```python
from build123d import *

# Parameters (mm, degrees)
BOSS_EXTRUDE1_DEPTH            = 3.175
M2X0_4_TAPPED_HOLE1_AT_2_COUNT = 2
M2X0_4_TAPPED_HOLE1_AT_2_PITCH = 18.662705418
CIRPATTERN1_COUNT              = 6


with BuildPart() as part:
    # Sketch1 → Boss-Extrude1 (new body)
    with BuildSketch(Plane(origin=(0, 0, 0), x_dir=(1, 0, 0), z_dir=(0, 1, 0))):
        Polygon((60.998522628, 0), (30.499261314, 52.826270189), (-30.499261314, 52.826270189), (-60.998522628, 0), (-30.499261314, -52.826270189), (30.499261314, -52.826270189), align=None)
        with BuildLine():
            Line((52.749630657, 1.5875), (27.749630657, 44.888770189))
            ThreePointArc((27.749630657, 44.888770189), (26.5875, 46.050900846), (25, 46.476270189))
            Line((25, 46.476270189), (-25, 46.476270189))
            ThreePointArc((-25, 46.476270189), (-26.5875, 46.050900846), (-27.749630657, 44.888770189))
            Line((-27.749630657, 44.888770189), (-52.749630657, 1.5875))
            ThreePointArc((-52.749630657, 1.5875), (-53.175, 0), (-52.749630657, -1.5875))
            Line((-52.749630657, -1.5875), (-27.749630657, -44.888770189))
            ThreePointArc((-27.749630657, -44.888770189), (-26.5875, -46.050900846), (-25, -46.476270189))
            Line((-25, -46.476270189), (25, -46.476270189))
            ThreePointArc((25, -46.476270189), (26.5875, -46.050900846), (27.749630657, -44.888770189))
            Line((27.749630657, -44.888770189), (52.749630657, -1.5875))
            ThreePointArc((52.749630657, -1.5875), (53.175, 0), (52.749630657, 1.5875))
        make_face(mode=Mode.SUBTRACT)
    extrude(amount=BOSS_EXTRUDE1_DEPTH)

    # Sketch2 → M2x0.4 Tapped Hole1 (revolve, cut)
    with BuildSketch(Plane(origin=(9.408369434, 3.175, -50.410234914), x_dir=(0, 0, 1), z_dir=(1, 0, 0))):
        Polygon((0, 0), (0, 6.576688495), (0.8, 6.096), (0.8, 0), align=None)
    m2x0_4_tapped_hole1 = revolve(axis=Axis((9.408369434, 9.525, -50.410234914), (0, -1, 0)), mode=Mode.SUBTRACT)

    # M2x0.4 Tapped Hole1 at 2: M2x0.4 Tapped Hole1 ×2
    with Locations(*[(-i * M2X0_4_TAPPED_HOLE1_AT_2_PITCH, 0, 0) for i in range(1, M2X0_4_TAPPED_HOLE1_AT_2_COUNT)]):
        add(m2x0_4_tapped_hole1, mode=Mode.SUBTRACT)

    # CirPattern1: M2x0.4 Tapped Hole1 ×6 about axis
    cirpattern1_axis = Axis((0, 0, 0), (0, 1, 0))
    for i in range(1, CIRPATTERN1_COUNT):
        add(m2x0_4_tapped_hole1.rotate(cirpattern1_axis, i * 360 / CIRPATTERN1_COUNT), mode=Mode.SUBTRACT)

    # CirPattern1 copy 1 sketch → CirPattern1 copy 1 (revolve, cut)
    with BuildSketch(Plane(origin=(-48.283712038, 3.175, -17.1906274), x_dir=(0.866025404, 0, 0.5), z_dir=(0.5, 0, -0.866025404))):
        Polygon((0, 0), (0, 6.576688495), (0.8, 6.096), (0.8, 0), align=None)
    revolve(axis=Axis((-48.283712038, 9.525, -17.1906274), (0, -1, 0)), mode=Mode.SUBTRACT)

    # CirPattern1 copy 2 sketch → CirPattern1 copy 2 (revolve, cut)
    with BuildSketch(Plane(origin=(-39.029376054, 3.175, 33.219607514), x_dir=(0.866025404, 0, -0.5), z_dir=(-0.5, 0, -0.866025404))):
        Polygon((0, 0), (0, 6.576688495), (0.8, 6.096), (0.8, 0), align=None)
    revolve(axis=Axis((-39.029376054, 9.525, 33.219607514), (0, -1, 0)), mode=Mode.SUBTRACT)

    # CirPattern1 copy 3 sketch → CirPattern1 copy 3 (revolve, cut)
    with BuildSketch(Plane(origin=(9.254335984, 3.175, 50.410234914), x_dir=(0, 0, -1), z_dir=(-1, 0, 0))):
        Polygon((0, 0), (0, 6.576688495), (0.8, 6.096), (0.8, 0), align=None)
    revolve(axis=Axis((9.254335984, 9.525, 50.410234914), (0, -1, 0)), mode=Mode.SUBTRACT)

    # CirPattern1 copy 4 sketch → CirPattern1 copy 4 (revolve, cut)
    with BuildSketch(Plane(origin=(48.283712038, 3.175, 17.1906274), x_dir=(-0.866025404, 0, -0.5), z_dir=(-0.5, 0, 0.866025404))):
        Polygon((0, 0), (0, 6.576688495), (0.8, 6.096), (0.8, 0), align=None)
    revolve(axis=Axis((48.283712038, 9.525, 17.1906274), (0, -1, 0)), mode=Mode.SUBTRACT)

    # CirPattern1 copy 5 sketch → CirPattern1 copy 5 (revolve, cut)
    with BuildSketch(Plane(origin=(39.029376054, 3.175, -33.219607514), x_dir=(-0.866025404, 0, 0.5), z_dir=(0.5, 0, 0.866025404))):
        Polygon((0, 0), (0, 6.576688495), (0.8, 6.096), (0.8, 0), align=None)
    revolve(axis=Axis((39.029376054, 9.525, -33.219607514), (0, -1, 0)), mode=Mode.SUBTRACT)


solid = part.part
```
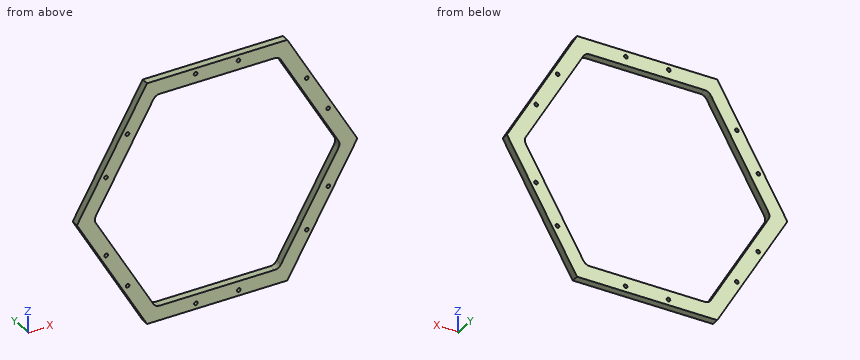
Verification items for the finished model (mm, model axes). Give positions to 0.01 mm unless a question says otherwise; leave off trailing zeros. Order: outer loops, then holes, each group sorted by start corner. A loop starts at its lowest first (then second) coordinate and runs counter-clockwise, first axis right, second up. Notation, with made-up numbers: M 89.25,-3.75 L 99.25,-3.75 A13 cw 99.25,20.25 Z; hole C -40,11.25 d7. An arc over 180 degrees is marked long. Answer in a Markdown table with one row per item. Add a question column.
Item 1: Gauge pin test, flat end, axial feed: pin 1 (1.8 mm diameter, centred on x = -38.95, z = -33.35, fed in from -Y). Record the tip position at first contact, or that the pin passes through.
Item 2: Section check B-B, the plane z = 37.5. Enter the section's corners in (x, y) (3 decimals), and give its area (3 significant figures).
Item 3: Section check C-C, the plane y = 0.75. State how many separate pieces and enclosed holes the cut face has, and give its area (3 significant figures).
Item 4: Scan lines: probe 1 along Z at (x, y) = (-5.5, 1.55); probe 2 along X at (y, z) = (2.8, 32.5); probe 3 along Z at (x, y) = (38, 2.45). Record each from-to range of solid material in increasing order. Write a range as from..to.
Item 5: Section check A-A, the plane x = -2.5. Enter the section's corners in (y, z) (3 decimals), and give its area (3 significant figures).
Filled sheet:
| question | item | result |
|---|---|---|
| 1 | pin 1 | stops at y = 0 |
| 2 | outline | M -39.348,0 L -32.016,0 L -32.016,3.175 L -39.348,3.175 Z; M 32.016,0 L 39.348,0 L 39.348,3.175 L 32.016,3.175 Z |
| 2 | area | 46.6 mm^2 |
| 3 | separate pieces | 1 |
| 3 | enclosed holes | 13 |
| 3 | area | 2,160 mm^2 |
| 4 | probe 1 | z = -52.83..-46.48, 46.48..52.83 |
| 4 | probe 2 | x = -42.23..-39.38, -38.68..-34.9, 34.9..42.23 |
| 4 | probe 3 | z = -39.83..-27.13, 27.13..39.83 |
| 5 | outline | M 0,-52.826 L 3.175,-52.826 L 3.175,-46.476 L 0,-46.476 Z; M 0,46.476 L 3.175,46.476 L 3.175,52.826 L 0,52.826 Z |
| 5 | area | 40.3 mm^2 |
